Work out the finished part from the listing and answer in its coordinate system (mm). A direction names the side the tool comes from. Give positions to 0.01 mm unless a question says otherwise; leave off trailing zeros. Write each loop counter-clockwise with the first axis right and the second up, starting at its lowest first coordinate (ties: lowest second). Pieces come first, ordered by that corner, then holes. Notation, with made-up numbers: (27, -3.5) -> (79, -3.5) arc R22 ccw to (79, 24.5) -> close; hole circle Ø4 at (10, 25). An arc over 180 degrees is marked (long way). Use a Markdown table: item, result. Add a question column.
Q1. For a pull along X with two mould halves and no side action, classify faces 3 (the face through (-20.486, 0.221, 2.712)), 4 (the face through (23.925, 0, 3)), 5 (the face through (17.114, 0.221, 2.712)), 6 (the face through (0, 0, 0)) as pulls with the +X half, pulls with the -X half, needs draft (parallel to the pull), parting line crosses it, or undercut.
Q2. For faces 1 (the face through (-23.925, 0, 3)), 2 (the face through (0, 0, 5.5)), determine the directions among +Z, -Z, +X, -X, +Y, -Y from which every point of the face is accessible in a straight line to the end or side of a thin tool.
Q3. Consider line 1 (X direction, y = 0, z = 2.75) (3 decimals); line 2 (Y direction, x = -18.8, z = 2.5) (3 decimals); line 3 (Y direction, x = 7.5, z = 6.25) (3 decimals). Determine where each line is inside the solid, lowest interval first.
Q4. This flat-tipped pin is pushed along its axis until it touches: pin 1 Ø2 at (x, y) = (-15, 1.5) entering from +Z. Where does it stop, or does it pass through?
Q5. Section A-A, the plane x = 18.8 is taken. Give the vertices of the cut face in (y, z) (3 decimals).
Q6. Section B-B, the plane z = 2.75 is taken. Give the vertices of the cut face in (x, y) (3 decimals).
Q7. Section D-D, the plane z = 6.75 is taken. Give the vertices of the cut face in (x, y) (3 decimals).
Q8. Section C-C, the plane y = 0 is taken. Give the vertices of the cut face in (x, z) (3 decimals), plus the area to 3 significant figures.
Autodesk Inventor part; units mm, degrees
ref_plane "YZ Plane" through (0, 0, 0) normal (1, 0, 0) x (0, 1, 0)
ref_plane "XZ Plane" through (0, 0, 0) normal (0, 1, 0) x (-1, 0, 0)
ref_plane "XY Plane" through (0, 0, 0) normal (0, 0, 1) x (1, 0, 0)
sketch "Sketch1" plane through (0, 0, 0) normal (0, 0, 1) x (1, 0, 0)
  line L0 (-23.925, -7.425) -> (23.925, -7.425)
  line L1 (23.925, -7.425) -> (23.925, 7.425)
  line L2 (23.925, 7.425) -> (-23.925, 7.425)
  line L3 (-23.925, 7.425) -> (-23.925, -7.425)
  line L4 (-23.925, -7.425) -> (23.925, 7.425) construction
  line L5 (23.925, -7.425) -> (-23.925, 7.425) construction
  point P0 (0, 0)
  dimension "d0" = 47.85
  dimension "d1" = 14.85
extrude "Extrusion1" add sketch "Sketch1" along normal blind 10.3
sketch "Sketch3" plane through (0, 0, 10.3) normal (0, 0, 1) x (1, 0, 0)
  line L0 (23.925, -7.425) -> (23.925, 7.425)
  line L1 (-23.925, 7.425) -> (-23.925, -7.425)
  line L2 (-23.925, -6.55) -> (23.925, -6.55)
  line L3 (23.925, -6.55) -> (23.925, 6.55)
  line L4 (23.925, 6.55) -> (-23.925, 6.55)
  line L5 (-23.925, 6.55) -> (-23.925, -6.55)
  line L6 (-23.925, -6.55) -> (23.925, 6.55) construction
  line L7 (23.925, -6.55) -> (-23.925, 6.55) construction
  point P0 (0, 0)
  dimension "d5" = 13.1
extrude "Extrusion2" cut sketch "Sketch3" against normal blind 4.8
sketch "Sketch4" plane through (0, 0, 5.5) normal (0, 0, 1) x (1, 0, 0)
  line L0 (-23.925, -6.55) -> (-23.925, 6.55) construction
  line L1 (-23.925, 0) -> (23.925, 0) construction
  line L2 (23.925, 6.55) -> (23.925, -6.55) construction
  point P0 (0, 0)
  point P1 (-18.8, 0)
  point P2 (18.8, 0)
  point P3 (0, 0)
  dimension "d8" = 18.8
  dimension "d9" = 18.8
hole "Hole1" at (-18.8, 0, 5.5) at (18.8, 0, 5.5) direction (0, 0, -1) diameter 3.4 end through all
equation "\"d0\" = sensorLength"
equation "\"d1\" = sensorWidth"
equation "\"d2\" = sensorDepth"
equation "\"d5\" = slotWidth"
equation "\"d6\" = slotDepth"
equation "\"sensorWidth\" = 14.85"
equation "\"sensorLength\" = 47.85"
equation "\"sensorDepth\" = 10.3"
equation "\"slotWidth\" = 13.1"
equation "\"slotDepth\" = 4.8"
equation "\"holeWidth\" = 37.6"
equation "\"holeDiameter\" = 3.4"
properties part number "sensor" material "Aluminum 6061"
Result set:
| question | item | result |
|---|---|---|
| 1 | face 3 | undercut |
| 1 | face 4 | pulls with the +X half |
| 1 | face 5 | undercut |
| 1 | face 6 | needs draft |
| 2 | face 1 | +Z, -Z, -X, +Y, -Y |
| 2 | face 2 | +Z, +X, -X |
| 3 | line 1 | x = -23.925 to -20.5, -17.1 to 17.1, 20.5 to 23.925 |
| 3 | line 2 | y = -7.425 to -1.7, 1.7 to 7.425 |
| 3 | line 3 | y = -7.425 to -6.55, 6.55 to 7.425 |
| 4 | pin 1 | stops at z = 5.5 |
| 5 | outline | (-7.425, 0) -> (-1.7, 0) -> (-1.7, 5.5) -> (-6.55, 5.5) -> (-6.55, 10.3) -> (-7.425, 10.3) -> close; (1.7, 0) -> (7.425, 0) -> (7.425, 10.3) -> (6.55, 10.3) -> (6.55, 5.5) -> (1.7, 5.5) -> close |
| 6 | outline | (-23.925, -7.425) -> (23.925, -7.425) -> (23.925, 7.425) -> (-23.925, 7.425) -> close; hole circle Ø3.4 at (-18.8, 0); hole circle Ø3.4 at (18.8, 0) |
| 7 | outline | (-23.925, -7.425) -> (23.925, -7.425) -> (23.925, -6.55) -> (-23.925, -6.55) -> close; (-23.925, 6.55) -> (23.925, 6.55) -> (23.925, 7.425) -> (-23.925, 7.425) -> close |
| 8 | outline | (-23.925, 0) -> (-20.5, 0) -> (-20.5, 5.5) -> (-23.925, 5.5) -> close; (-17.1, 0) -> (17.1, 0) -> (17.1, 5.5) -> (-17.1, 5.5) -> close; (20.5, 0) -> (23.925, 0) -> (23.925, 5.5) -> (20.5, 5.5) -> close |
| 8 | area | 226 mm2 |
